Autodesk Inventor part; units mm, degrees
ref_plane "YZ Plane" through (0, 0, 0) normal (1, 0, 0) x (0, 1, 0)
ref_plane "XZ Plane" through (0, 0, 0) normal (0, 1, 0) x (-1, 0, 0)
ref_plane "XY Plane" through (0, 0, 0) normal (0, 0, 1) x (1, 0, 0)
sketch "Sketch1" plane through (0, 0, 0) normal (0, 1, 0) x (-1, 0, 0)
  line L0 (20, 22.5) -> (-20, 22.5)
  line L1 (-20, 22.5) -> (-20, -100)
  line L2 (-20, -100) -> (20, -100)
  line L3 (20, -100) -> (20, 22.5)
  circle A0 centre (0, 0) radius 4
  dimension "d0" = 122.5
  dimension "d1" = 22.5
  dimension "d2" = 40
  dimension "d3" = 20
  dimension "d4" = 8
extrude "Extrusion1" add sketch "Sketch1" along normal blind 5
sketch "Sketch2" plane through (0, 5, 0) normal (0, 1, 0) x (1, 0, 0)
  line L0 (-20, 100) -> (-20, -22.5)
  line L1 (20, -22.5) -> (20, 100)
  line L2 (-20, -22.5) -> (20, -22.5)
  line L3 (20, -22.5) -> (20, 100)
  line L4 (20, 100) -> (-20, 100)
  line L5 (-20, 100) -> (-20, -22.5)
  line L6 (-15, -17.5) -> (15, -17.5)
  line L7 (15, -17.5) -> (15, 95)
  line L8 (15, 95) -> (-15, 95)
  line L9 (-15, 95) -> (-15, -17.5)
  point P0 (0, 0)
  dimension "d7" = 5
  dimension "d8" = 5
  dimension "d9" = 5
  dimension "d10" = 5
extrude "Extrusion2" add sketch "Sketch2" along normal blind 35
sketch "Sketch3" plane through (0, 40, 0) normal (0, 1, 0) x (1, 0, 0)
  line L0 (-20, 100) -> (-20, -22.5)
  line L1 (20, -22.5) -> (20, 100)
  line L2 (-20, 100) -> (20, 100)
  line L3 (20, 100) -> (20, 22.5)
  line L4 (20, 22.5) -> (-20, 22.5)
  line L5 (-20, 22.5) -> (-20, 100)
  point P0 (0, 0)
  point P1 (-20, 22.5)
  dimension "d13" = 77.5
extrude "Extrusion3" add sketch "Sketch3" against normal blind 5
sketch "Sketch4" plane through (0, 5, 0) normal (0, 1, 0) x (1, 0, 0)
  line L0 (-15, -17.5) -> (-15, 22.5)
  line L1 (15, 22.5) -> (15, -17.5)
  line L2 (-15, -17.5) -> (15, -17.5)
  line L3 (15, -17.5) -> (15, 17.5)
  line L4 (15, 17.5) -> (-15, 17.5)
  line L5 (-15, 17.5) -> (-15, -17.5)
  point P0 (0, 0)
  point P1 (-15, 17.5)
  dimension "d16" = 35
extrude "Extrusion4" add sketch "Sketch4" along normal blind 20
sketch "Sketch5" plane through (0, 0, 0) normal (0, -1, 0) x (1, 0, 0)
  circle A0 centre (0, 0) radius 4
  circle A1 centre (0, 0) radius 9.5
  dimension "d19" = 19
extrude "Extrusion5" cut sketch "Sketch5" against normal blind 12.5 contours A0 | A1
sketch "Sketch6" plane through (0, 0, 0) normal (0, -1, 0) x (1, 0, 0)
  circle A0 centre (0, 0) radius 11.5
  dimension "d22" = 23
extrude "Extrusion6" cut sketch "Sketch6" against normal blind 6.5
sketch "Sketch7" plane through (0, 12.5, 0) normal (0, -1, 0) x (1, 0, 0)
  circle A0 centre (0, 0) radius 9.5
  circle A1 centre (0, 0) radius 6.2
  line L0 (0, 0) -> (0, 7.0938)
  line L1 (0, 0) -> (7.0405, -4.0648)
  line L2 (0, 0) -> (-6.9896, -4.0354)
  circle A2 centre (0, 6.2) radius 1.45
  circle A3 centre (5.3694, -3.1) radius 1.45
  circle A4 centre (-5.3694, -3.1) radius 1.45
  dimension "d25" = 12.4
  dimension "d26" = 120
  dimension "d27" = 120
  dimension "d28" = 2.9
  dimension "d29" = 2.9
  dimension "d30" = 2.9
extrude "Extrusion7" cut sketch "Sketch7" against normal blind 18 contours A2 L0 A1 | A1 A2 | A3 L1 A1 | A1 L1 A3 | L0 A2 A1 | L1 A3 A1 | A1 A3 L1 | A4 L2 A1 | A1 L2 A4 | A4 A1 L2 | A4 L2 A1
sketch "Sketch8" plane through (0, 0, 0) normal (0, -1, 0) x (1, 0, 0)
  line L0 (15, -95) -> (-15, -95)
  line L1 (-15, -95) -> (-15, -22.5)
  line L2 (15, -95) -> (-15, -95)
  line L3 (-15, -95) -> (-15, -17.5)
  line L4 (-15, -17.5) -> (15, -17.5)
  line L5 (15, -17.5) -> (15, -95)
  point P0 (0, 0)
  dimension "d33" = 77.5
extrude "Extrusion8" cut sketch "Sketch8" against normal blind 18
sketch "Sketch9" plane through (-15, 0, -95) normal (0, 0, 1) x (1, 0, 0)
  line L0 (30, 35) -> (0, 35)
  line L1 (30, 35) -> (0, 35)
  line L2 (0, 35) -> (0, 0)
  line L3 (0, 0) -> (30, 0)
  line L4 (30, 0) -> (30, 35)
  point P0 (15, 0)
extrude "Extrusion9" add sketch "Sketch9" along normal blind 3
sketch "Sketch10" plane through (20, 0, -100) normal (0, 0, -1) x (-1, 0, 0)
  circle A0 centre (20, 20) radius 4
  line L0 (0, 0) -> (0, 40)
  line L1 (0, 0) -> (40, 0)
  line L2 (35, 35) -> (5, 35)
  line L3 (20, 35) -> (20, 7.5388)
  circle A1 centre (20, 20) radius 8.5
  circle A2 centre (20, 11.5) radius 1.5
  circle A3 centre (20, 28.5) radius 1.5
  point P0 (20, 0)
  dimension "d38" = 20
  dimension "d39" = 20
  dimension "d40" = 8
  dimension "d41" = 17
  dimension "d42" = 3
  dimension "d43" = 3
extrude "Extrusion10" cut sketch "Sketch10" against normal blind 9 contours A0 L3 | L3 A0 | A3 A1 L3 | L3 A1 A3 | A2 A1 L3 | L3 A1 A2 | A1 A3 L3 | L3 A3 A1 | A1 A2 L3 | L3 A2 A1
fillet "Fillet1" radius 2 4 edges at (-20, 20, 22.5) (20, 20, 22.5) (20, 20, -100) (-20, 20, -100)
fillet "Fillet2" radius 2 2 edges at (15, 12.5, -17.5) (-15, 12.5, -17.5)
fillet "Fillet3" radius 2 2 edges at (-15, 37.5, -22.5) (15, 37.5, -22.5)
sketch "Sketch11" plane through (-15, 0, -92) normal (0, 0, 1) x (1, 0, 0)
  circle A0 centre (15, 20) radius 4
  circle A1 centre (15, 20) radius 13
  point P0 (15, 0)
  dimension "d49" = 26
extrude "Extrusion11" cut sketch "Sketch11" against normal blind 4
properties part number "Link6_v2"
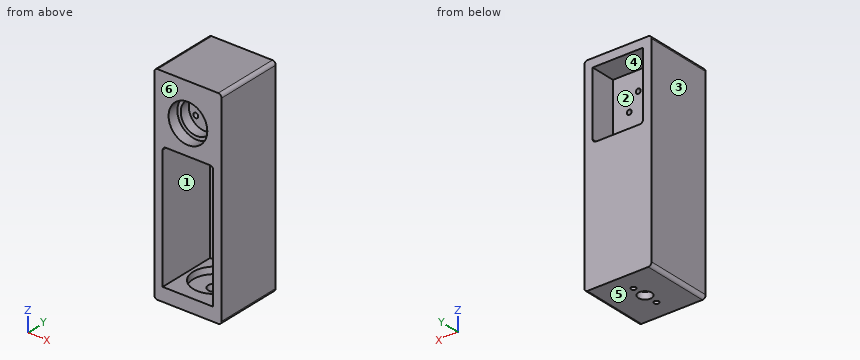
Can you work these out from the model? Positions are in its coordinate system, mm. Face numbers are marked on the shaded views. A direction names the side the tool comes from. Give positions to 0.01 mm unless a question says otherwise; leave off trailing zeros. Loops run counter-clockwise (first coordinate to the right, second up) from the corner with the lowest first, then second, coordinate; pieces in that order, holes last. Notation, with made-up numbers: (61.25, -6) - (115.25, -6) arc R21 cw to (115.25, 4) - close; hole circle Ø9 at (8.25, 53). An arc over 180 degrees is marked (long way). Return JSON: item names as keys, results as strings.
1. I'm going to push flat-ended pins straight in: pin 1 Ø4 at (x, z) = (-15.5, -42) entering from -Y; pin 2 Ø3.5 at (x, z) = (-5.37, -3.1) entering from -Y; pin 3 Ø4.5 at (x, z) = (5.37, -3.1) entering from +Y. Where does each tip first touch, or does it pass through?
Output values:
{"pin 1": "stops at y = 0", "pin 2": "stops at y = 12.5", "pin 3": "stops at y = 25"}
2. I want a section at D-D on y = 28.5. Please give me the cut outline in (x, z), and give its area (3 significant figures).
Output values:
{"outline": "(-20, -98) arc R2 ccw to (-18, -100) - (-1.5, -100) - (-1.5, -96) - (-9.84, -96) - (-9.84, -92) - (-15, -92) - (-15, 17.5) - (15, 17.5) - (15, -92) - (9.84, -92) - (9.84, -96) - (1.5, -96) - (1.5, -100) - (18, -100) arc R2 ccw to (20, -98) - (20, 20.5) arc R2 ccw to (18, 22.5) - (-18, 22.5) arc R2 ccw to (-20, 20.5) - close", "area": "1,520 mm²"}
3. I want a section at B-B on z = 6.2. Please give me the cut outline in (x, y).
Output values:
{"outline": "(-20, 0) - (-9.69, 0) - (-9.69, 6.5) - (-7.2, 6.5) - (-7.2, 12.5) - (-1.45, 12.5) - (-1.45, 25) - (-15, 25) - (-15, 40) - (-20, 40) - close; (1.45, 12.5) - (7.2, 12.5) - (7.2, 6.5) - (9.69, 6.5) - (9.69, 0) - (20, 0) - (20, 40) - (15, 40) - (15, 25) - (1.45, 25) - close"}
4. If I drill on line 1 (Y direction, x = 0, z = -97.8); line 2 (Z direction, x = 0, y = 2.25); line 3 (X direction, y = 17, z = 6), over which ranges is the centre line in solid material (lowest first)?
Output values:
{"line 1": "y = 0 to 10, 13 to 16, 24 to 27, 30 to 40", "line 2": "z = -100 to -92, -17.5 to -11.5, 11.5 to 22.5", "line 3": "x = -20 to -1.44, 1.44 to 20"}
5. I want a section at A-A on y = 20. Please give me the cut outline in (x, z), and give its area (3 significant figures).
Output values:
{"outline": "(-20, -98) arc R2 ccw to (-18, -100) - (-4, -100) - (-4, -96) - (-13, -96) - (-13, -92) - (-15, -92) - (-15, -19.5) arc R2 cw to (-13, -17.5) - (13, -17.5) arc R2 cw to (15, -19.5) - (15, -92) - (13, -92) - (13, -96) - (4, -96) - (4, -100) - (18, -100) arc R2 ccw to (20, -98) - (20, 20.5) arc R2 ccw to (18, 22.5) - (-18, 22.5) arc R2 ccw to (-20, 20.5) - close; hole circle Ø2.9 at (-5.37, -3.1); hole circle Ø2.9 at (0, 6.2); hole circle Ø2.9 at (5.37, -3.1)", "area": "2,510 mm²"}
6. I want a section at C-C on z = -59. Please give me the cut outline in (x, y).
Output values:
{"outline": "(-20, 0) - (-15, 0) - (-15, 35) - (15, 35) - (15, 0) - (20, 0) - (20, 40) - (-20, 40) - close"}
7. For the marked faces 1, 2 and 3, which set-ups out of +Z, -Z, +X, -X, +Y, -Y let a thin tool reach every point of the face, with its end or its side?
Output values:
{"face 1": "none", "face 2": "+Y", "face 3": "+Z, -Z, -X, +Y, -Y"}
8. We'd pull the mould along Z, two halves only. Please class the marked faces 4, 5 and 6: +Z half, -Z half, draft (parallel to the pull), parting line (faces both ways), or undercut.
Output values:
{"face 4": "undercut", "face 5": "-Z half", "face 6": "draft"}
